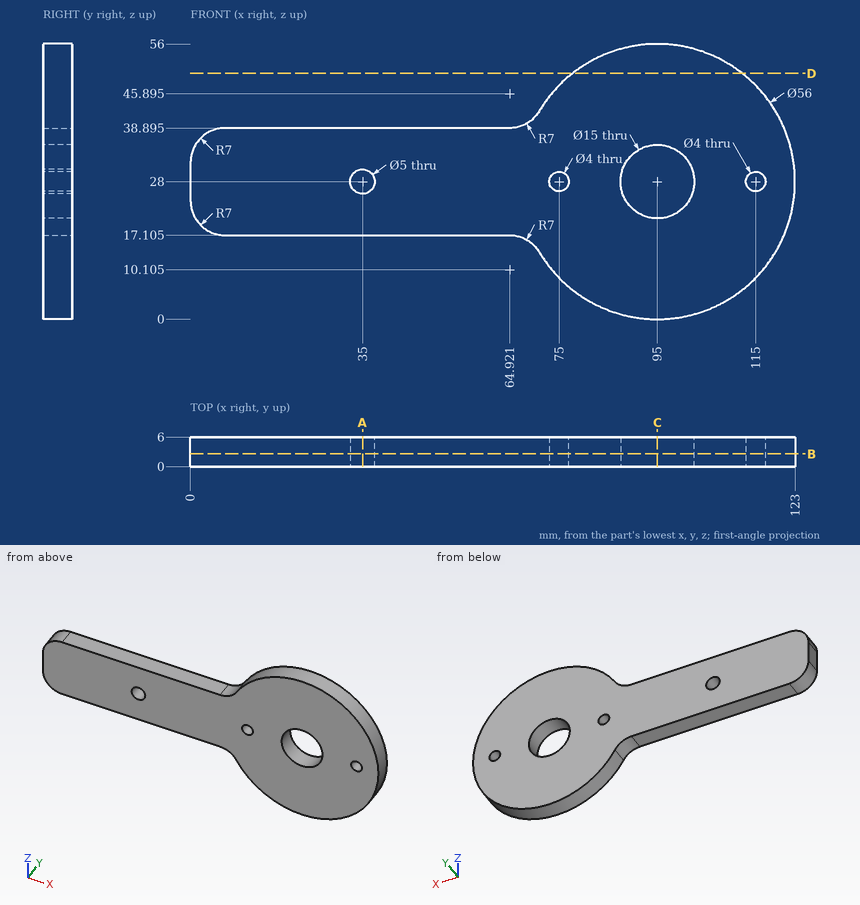
Geometry check sheet. Reference: drawing and pictorial views, mm from the part's lowest x, y, z. Coordinates: 2 decimals unless noted, no trailing zeros. Write each loop counter-clockwise with the first axis right and the second up, starting at its lowest first coordinate (ties: lowest second). Pieces come first, ordered by that corner, then holes. Notation, with made-up numbers: (1, 57.5) - (9, 57.5) arc R26 cw to (9, 94.5) - close; hole circle Ø8 at (-34.5, -4). An arc over 180 degrees is marked (long way). Write item = value, one per line.
Q1. Go/stop test with flat-tipped pins: pin 1 Ø2.5 at (x, z) = (75, 28) entering from +Y; pin 2 Ø1.5 at (y, z) = (1, 11.5) entering from +X; pin 3 Ø1.5 at (y, z) = (1.5, 34.5) entering from -X; pin 4 Ø1 at (y, z) = (0.5, 30.5) entering from +X. Record where each tip stops, or that it passes through.
Answer:
pin_1 = through
pin_2 = 118.15
pin_3 = 0.25
pin_4 = 122.93
Q2. Cross-section at B-B (y = 2.6). Enter the section's corners in (x, z) (1 decimal).
Answer:
outline = (0, 24.1) arc R7 ccw to (7, 17.1) - (64.9, 17.1) arc R7 cw to (70.9, 13.7) arc R28 ccw (long way) to (70.9, 42.3) arc R7 cw to (64.9, 38.9) - (7, 38.9) arc R7 ccw to (0, 31.9) - close; hole circle Ø5 at (35, 28); hole circle Ø4 at (75, 28); hole circle Ø15 at (95, 28); hole circle Ø4 at (115, 28)
Q3. Cross-section at C-C (x = 95). Enter the section's corners in (y, z), plus the area to 3 significant figures.
Answer:
outline = (0, 0) - (6, 0) - (6, 20.5) - (0, 20.5) - close; (0, 35.5) - (6, 35.5) - (6, 56) - (0, 56) - close
area = 246 mm²
Q4. Cross-section at A-A (x = 35). Enter the section's corners in (y, z) (1 decimal).
Answer:
outline = (0, 17.1) - (6, 17.1) - (6, 25.5) - (0, 25.5) - close; (0, 30.5) - (6, 30.5) - (6, 38.9) - (0, 38.9) - close
Q5. Cross-section at D-D (z = 50). Enter the section's corners in (x, y), plus the area to 3 significant figures.
Answer:
outline = (77.68, 0) - (112.32, 0) - (112.32, 6) - (77.68, 6) - close
area = 208 mm²
Q6. Material ranges on L1, parallel to X at y = 0.35, z = 29; L2, parallel to Z at x = 95, y = 4.35; L3, parallel to Z at x = 35, y = 4.7 (1 decimal), recorded low to high. Write a range as from..to.
Answer:
L1 = 0..32.71, 37.29..73.27, 76.73..87.57, 102.43..113.27, 116.73..122.98
L2 = 0..20.5, 35.5..56
L3 = 17.1..25.5, 30.5..38.9
